Geometry: final body of the model. Coordinates: model frame, mm. Face numbers are marked on the shaded views. A direction names the side the tool comes from. Give positions to 0.01 mm unless a question says otherwise; leave off trailing zeros. Write each loop counter-clockwise with the first axis right and the second up, starting at its lowest first coordinate (ties: lowest second). Pieces come first, ordered by that corner, then holes. Notation, with made-up numbers: (16.5, 84) -> (62.5, 84) arc R31 cw to (62.5, 122) -> close; hole circle Ø5 at (-3, -38). An arc over 180 degrees is marked (long way). Answer in a Markdown table with one row per item. Add a question column.
Item 1: Section query C-C on y = 2. State how many separate pieces and enclosed holes the cut face has, plus the area to 3 significant figures.
Item 2: Draft query along Z for the marked faces 3, 4, 5 and 6. Return one class per face: +Z half, -Z half, draft (parallel to the pull), parting line (faces both ways), or undercut.
Item 3: Section query D-D on z = -2.5. Output: boundary loops of the cut face in (x, y), plus the area to 3 significant figures.
Item 4: Material intervals for probe 1 along Z at (x, y) = (1.5, -7.5); probe 2 along Z at (x, y) = (3.25, -2.5); probe 3 along X at (y, z) = (-3.5, -13.5), sorted ascending. Write a range as from..to.
Item 5: First-contact query: P1, Ø4.5, axis at x = 18, z = -8, coming from the -Y side; P2, Ø6, axis at x = 11.5, z = -8, coming from the +Y side; P3, Ø0.9, axis at x = 1.5, z = -13.5, coming from the +Y side; P4, Ø2, axis at y = -4.5, z = -2.5, coming from the +X side. Flat tips, straight axial feed; report the tip coordinate or a pass-through.
Item 6: Access query for the marked faces 1 and 2. Directions: +Z, -Z, +X, -X, +Y, -Y. A direction counts if a zero-diameter tool reaches every point of the face in a straight line with its end or side. Return the directions, or none.
Item 7: Section query A-A on y = -3. Output: boundary loops of the cut face in (x, z), plus the area to 3 significant figures.
Item 8: Section query B-B on z = -5.88. Output: boundary loops of the cut face in (x, y).
```python
from build123d import *

# Parameters (mm, degrees)
ESQUISSE1_W             = 29
ESQUISSE1_H             = 15
BOSS_EXTRU_1_DEPTH      = 1
ESQUISSE2_R             = 1.016
BOSS_EXTRU_2_DEPTH      = 2
BOSS_EXTRU_2_DEPTH_BACK = 12
CHANFREIN1_SIZE         = 1.5
CHANFREIN1_SIZE2        = 0.6
CHANFREIN1_PART_2_SIZE  = 1.5
CHANFREIN1_PART_2_SIZE2 = 0.6
CHANFREIN1_PART_3_SIZE  = 1.5
CHANFREIN1_PART_3_SIZE2 = 0.6
CHANFREIN1_PART_4_SIZE  = 1.5
CHANFREIN1_PART_4_SIZE2 = 0.6
CHANFREIN1_PART_5_SIZE  = 1.5
CHANFREIN1_PART_5_SIZE2 = 0.6
CHANFREIN1_PART_6_SIZE  = 1.5
CHANFREIN1_PART_6_SIZE2 = 0.6
CHANFREIN1_PART_7_SIZE  = 1.5
CHANFREIN1_PART_7_SIZE2 = 0.6
CHANFREIN1_PART_8_SIZE  = 1.5
CHANFREIN1_PART_8_SIZE2 = 0.6
BOSS_EXTRU_3_DEPTH      = 3
CONG_2_R                = 0.5
CONG_3_R                = 0.5


with BuildPart() as part:
    # Esquisse1 → Boss.-Extru.1 (new body)
    with BuildSketch(Plane(origin=(0, 0, 0), x_dir=(1, 0, 0), z_dir=(0, 1, 0))):
        with Locations((14.5, 7.5)):
            Rectangle(ESQUISSE1_W, ESQUISSE1_H)
    extrude(amount=BOSS_EXTRU_1_DEPTH)

    # Esquisse2 → Boss.-Extru.2 (add, two sides)
    with BuildSketch(Plane(origin=(0, 1, 0), x_dir=(1, 0, 0), z_dir=(0, 1, 0))) as boss_extru_2_sk:
        with Locations((1.5, 13.5)):
            Circle(ESQUISSE2_R)
        with Locations((1.5, 10.96)):
            Circle(ESQUISSE2_R)
        with Locations((1.5, 8.42)):
            Circle(ESQUISSE2_R)
        with Locations((1.5, 5.88)):
            Circle(ESQUISSE2_R)
        with Locations((4.04, 10.96)):
            Circle(ESQUISSE2_R)
        with Locations((4.04, 8.42)):
            Circle(ESQUISSE2_R)
        with Locations((4.04, 5.88)):
            Circle(ESQUISSE2_R)
        with Locations((4.04, 13.5)):
            Circle(ESQUISSE2_R)
    extrude(amount=BOSS_EXTRU_2_DEPTH)
    extrude(boss_extru_2_sk.sketch, amount=-BOSS_EXTRU_2_DEPTH_BACK)

    # Chanfrein1
    chanfrein1_edges = [part.edges().sort_by_distance(p)[0] for p in [
        (0.484, 3, -13.5),
    ]]
    chanfrein1_side = [part.faces().sort_by_distance(p)[0] for p in [
        (0.484, 2, -13.5),
    ]]
    chamfer(chanfrein1_edges, length=CHANFREIN1_SIZE, length2=CHANFREIN1_SIZE2, reference=chanfrein1_side[0])

    # Chanfrein1 part 2
    chanfrein1_part_2_edges = [part.edges().sort_by_distance(p)[0] for p in [
        (0.484, 3, -10.96),
    ]]
    chanfrein1_part_2_side = [part.faces().sort_by_distance(p)[0] for p in [
        (0.484, 2, -10.96),
    ]]
    chamfer(chanfrein1_part_2_edges, length=CHANFREIN1_PART_2_SIZE, length2=CHANFREIN1_PART_2_SIZE2, reference=chanfrein1_part_2_side[0])

    # Chanfrein1 part 3
    chanfrein1_part_3_edges = [part.edges().sort_by_distance(p)[0] for p in [
        (0.484, 3, -8.42),
    ]]
    chanfrein1_part_3_side = [part.faces().sort_by_distance(p)[0] for p in [
        (0.484, 2, -8.42),
    ]]
    chamfer(chanfrein1_part_3_edges, length=CHANFREIN1_PART_3_SIZE, length2=CHANFREIN1_PART_3_SIZE2, reference=chanfrein1_part_3_side[0])

    # Chanfrein1 part 4
    chanfrein1_part_4_edges = [part.edges().sort_by_distance(p)[0] for p in [
        (0.484, 3, -5.88),
    ]]
    chanfrein1_part_4_side = [part.faces().sort_by_distance(p)[0] for p in [
        (0.484, 2, -5.88),
    ]]
    chamfer(chanfrein1_part_4_edges, length=CHANFREIN1_PART_4_SIZE, length2=CHANFREIN1_PART_4_SIZE2, reference=chanfrein1_part_4_side[0])

    # Chanfrein1 part 5
    chanfrein1_part_5_edges = [part.edges().sort_by_distance(p)[0] for p in [
        (3.024, 3, -10.96),
    ]]
    chanfrein1_part_5_side = [part.faces().sort_by_distance(p)[0] for p in [
        (3.024, 2, -10.96),
    ]]
    chamfer(chanfrein1_part_5_edges, length=CHANFREIN1_PART_5_SIZE, length2=CHANFREIN1_PART_5_SIZE2, reference=chanfrein1_part_5_side[0])

    # Chanfrein1 part 6
    chanfrein1_part_6_edges = [part.edges().sort_by_distance(p)[0] for p in [
        (3.024, 3, -8.42),
    ]]
    chanfrein1_part_6_side = [part.faces().sort_by_distance(p)[0] for p in [
        (3.024, 2, -8.42),
    ]]
    chamfer(chanfrein1_part_6_edges, length=CHANFREIN1_PART_6_SIZE, length2=CHANFREIN1_PART_6_SIZE2, reference=chanfrein1_part_6_side[0])

    # Chanfrein1 part 7
    chanfrein1_part_7_edges = [part.edges().sort_by_distance(p)[0] for p in [
        (3.024, 3, -5.88),
    ]]
    chanfrein1_part_7_side = [part.faces().sort_by_distance(p)[0] for p in [
        (3.024, 2, -5.88),
    ]]
    chamfer(chanfrein1_part_7_edges, length=CHANFREIN1_PART_7_SIZE, length2=CHANFREIN1_PART_7_SIZE2, reference=chanfrein1_part_7_side[0])

    # Chanfrein1 part 8
    chanfrein1_part_8_edges = [part.edges().sort_by_distance(p)[0] for p in [
        (3.024, 3, -13.5),
    ]]
    chanfrein1_part_8_side = [part.faces().sort_by_distance(p)[0] for p in [
        (3.024, 2, -13.5),
    ]]
    chamfer(chanfrein1_part_8_edges, length=CHANFREIN1_PART_8_SIZE, length2=CHANFREIN1_PART_8_SIZE2, reference=chanfrein1_part_8_side[0])

    # Esquisse3 → Boss.-Extru.3 (add)
    with BuildSketch(Plane(origin=(0, 1, 0), x_dir=(1, 0, 0), z_dir=(0, 1, 0))):
        with BuildLine():
            Line((7, 4), (18.771127801, 4))
            ThreePointArc((18.771127801, 4), (20.271127801, 2.5), (18.771127801, 1))
            Line((18.771127801, 1), (7, 1))
            ThreePointArc((7, 1), (5.5, 2.5), (7, 4))
        make_face()
    extrude(amount=BOSS_EXTRU_3_DEPTH)

    # Congé2
    cong_2_edges = [part.edges().sort_by_distance(p)[0] for p in [
        (5.5, 4, -2.5),
        (12.885563901, 4, -1),
        (20.271127801, 4, -2.5),
        (12.885563901, 4, -4),
    ]]
    fillet(cong_2_edges, radius=CONG_2_R)

    # Congé3
    cong_3_edges = [part.edges().sort_by_distance(p)[0] for p in [
        (5.5, 1, -2.5),
        (12.885563901, 1, -1),
        (20.271127801, 1, -2.5),
        (12.885563901, 1, -4),
    ]]
    fillet(cong_3_edges, radius=CONG_3_R)


solid = part.part
```
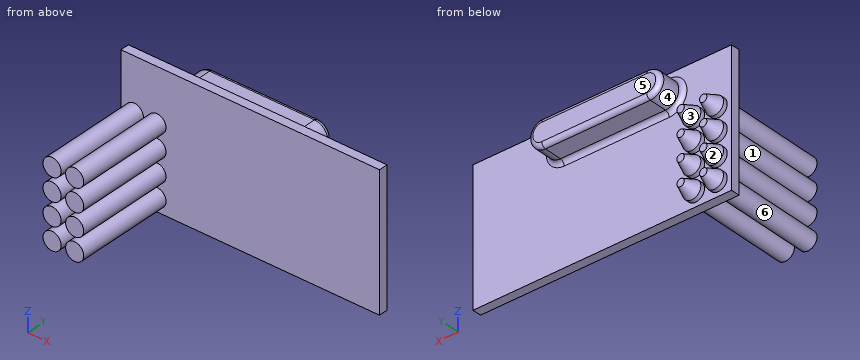
Findings below:
| question | item | result |
|---|---|---|
| 1 | separate pieces | 9 |
| 1 | enclosed holes | 0 |
| 1 | area | 59.1 mm^2 |
| 2 | face 3 | undercut |
| 2 | face 4 | parting line |
| 2 | face 5 | draft |
| 2 | face 6 | undercut |
| 3 | outline | (0, 0) -> (29, 0) -> (29, 1) -> (20.77, 1) arc R0.5 cw to (20.27, 1.5) -> (20.27, 3.5) arc R0.5 ccw to (19.77, 4) -> (6, 4) arc R0.5 ccw to (5.5, 3.5) -> (5.5, 1.5) arc R0.5 cw to (5, 1) -> (0, 1) -> close |
| 3 | area | 73.3 mm^2 |
| 4 | probe 1 | z = -14.52..-12.48, -11.98..-9.94, -9.44..-7.4, -6.9..-4.86 |
| 4 | probe 2 | z = -14.14..-12.86, -11.6..-10.32, -9.06..-7.78, -6.52..-5.24 |
| 4 | probe 3 | x = 0.48..2.52, 3.02..5.06 |
| 5 | P1 | stops at y = 0 |
| 5 | P2 | stops at y = 1 |
| 5 | P3 | stops at y = 3 |
| 5 | P4 | passes through |
| 6 | face 1 | -Y |
| 6 | face 2 | +Y |
| 7 | outline | circle Ø2.03 at (1.5, -13.5); circle Ø2.03 at (1.5, -10.96); circle Ø2.03 at (1.5, -8.42); circle Ø2.03 at (1.5, -5.88); circle Ø2.03 at (4.04, -13.5); circle Ø2.03 at (4.04, -10.96); circle Ø2.03 at (4.04, -8.42); circle Ø2.03 at (4.04, -5.88) |
| 7 | area | 25.9 mm^2 |
| 8 | outline | (0, 0) -> (0.48, 0) -> (0.48, -11) -> (2.52, -11) -> (2.52, 0) -> (3.02, 0) -> (3.02, -11) -> (5.06, -11) -> (5.06, 0) -> (29, 0) -> (29, 1) -> (5.06, 1) -> (5.06, 1.5) -> (4.46, 3) -> (3.62, 3) -> (3.02, 1.5) -> (3.02, 1) -> (2.52, 1) -> (2.52, 1.5) -> (1.92, 3) -> (1.08, 3) -> (0.48, 1.5) -> (0.48, 1) -> (0, 1) -> close |
